```python
from build123d import *

# Parameters (mm, degrees)
F0_W     = 25.4
F0_H     = 38.1
F1_DEPTH = 31.75
F2_W     = 6.223
F2_H     = 31.75
F3_DEPTH = 38.1
F4_R     = 6.6675
F5_DEPTH = 31.751
F6_R     = 1.905
F7_DEPTH = 38.101


with BuildPart() as f1:
    # F0 (on Top) → F1 (new body)
    with BuildSketch(Plane.XY):
        Rectangle(F0_W, F0_H)
    extrude(amount=F1_DEPTH)

    # F2 (on face) → F3 (join)
    with BuildSketch(Plane.YZ.offset(12.7)):
        with Locations((-15.9385, 15.875)):
            Rectangle(F2_W, F2_H)
        with Locations((15.9385, 15.875)):
            Rectangle(F2_W, F2_H)
    extrude(amount=F3_DEPTH)

    # F4 (on face) → F5 (cut, through all)
    with BuildSketch(Plane.XY.offset(31.75)):
        Circle(F4_R)
    extrude(amount=-F5_DEPTH, mode=Mode.SUBTRACT)

    # F6 (on face) → F7 (cut, through all)
    with BuildSketch(Plane(origin=(0, 19.05, 0), x_dir=(-1, 0, 0), z_dir=(0, 1, 0))):
        with Locations((-45.24375, 15.875)):
            Circle(F6_R)
        with Locations((-18.25625, 15.875)):
            Circle(F6_R)
    extrude(amount=-F7_DEPTH, mode=Mode.SUBTRACT)


solid = f1.part
```
Check sheet for the modelled part. Datum: model origin and axes. Units: mm. A direction names the side the tool comes from. Coordinates: 2 decimals unless noted, no trailing zeros. Loops run counter-clockwise (first coordinate to the right, second up) from the corner with the lowest first, then second, coordinate; pieces in that order, holes last.
1) Access from +Z, -Z, +X, -X, +Y, -Y to the whole of each face (thin tool, end or side, straight path). Record for faces 1 (the face through (12, 0, 31.75)), 2 (the face through (31, 12.827, 16)).
2) Sectioned sample at A-A (y = 0). Record the boundary of the cut face in (x, z).
3) Sectioned sample at C-C (z = 15). Count the separate pieces of the cut face and the enclosed holes in it, and give its area (3 significant figures).
4) Material ranges on probe 1 along Y at (x, z) = (0, 23.5); probe 2 along Y at (x, z) = (47, 9); probe 3 along X at (y, z) = (10.5, 20), recorded low to high.
5) Gauge pin test, flat end, axial feed: pin 1 (6 mm diameter, centred on y = 7, z = 7.5, fed in from +X). Record the tip position at first contact, or that the pin passes through.
6) Release check for a two-part mould opening along X. For faces 3 (the face through (-0.87, 6.61, 16.1)), 4 (the face through (31, -12.827, 16)), 5 (the face through (-12.7, 0, 16)) record: released by +X, released by -X, zero draft, split by the parting line, or undercut.
7) Sectioned sample at B-B (x = 0). Record the boundary of the cut face in (y, z).
8) Sectioned sample at D-D (x = 46). Record the boundary of the cut face in (y, z), and give its area (3 significant figures).
Check sheet entries:
1. face 1: +Z, +X, -X, +Y, -Y
1. face 2: +Z, -Z, +X
2. outline: (-12.7, 0) - (-6.67, 0) - (-6.67, 31.75) - (-12.7, 31.75) - close; (6.67, 0) - (12.7, 0) - (12.7, 31.75) - (6.67, 31.75) - close
3. separate pieces: 5
3. enclosed holes: 1
3. area: 1,220 mm2
4. probe 1: y = -19.05 to -6.67, 6.67 to 19.05
4. probe 2: y = -19.05 to -12.83, 12.83 to 19.05
4. probe 3: x = -12.7 to 12.7
5. pin 1: stops at x = 12.7
6. face 3: undercut
6. face 4: zero draft
6. face 5: released by -X
7. outline: (-19.05, 0) - (-6.67, 0) - (-6.67, 31.75) - (-19.05, 31.75) - close; (6.67, 0) - (19.05, 0) - (19.05, 31.75) - (6.67, 31.75) - close
8. outline: (-19.05, 0) - (-12.83, 0) - (-12.83, 14.13) - (-19.05, 14.13) - close; (-19.05, 17.62) - (-12.83, 17.62) - (-12.83, 31.75) - (-19.05, 31.75) - close; (12.83, 0) - (19.05, 0) - (19.05, 14.13) - (12.83, 14.13) - close; (12.83, 17.62) - (19.05, 17.62) - (19.05, 31.75) - (12.83, 31.75) - close
8. area: 352 mm2
